```python
from build123d import *

# Parameters (mm, degrees)
SKETCH1_R                = 4
BOSS_EXTRUDE1_DEPTH      = 5
BOSS_EXTRUDE2_DEPTH      = 50
BOSS_EXTRUDE2_DEPTH_BACK = 55
SKETCH2_W                = 150
SKETCH2_H                = 5
FILLET1_R                = 25


with BuildPart() as part:
    # Sketch1 → Boss-Extrude1 (new body)
    with BuildSketch(Plane.XY):
        with BuildLine():
            Line((-366.666725266, 12.5), (-126.666725266, 12.5))
            Line((-126.666725266, 12.5), (53.333274734, 12.5))
            ThreePointArc((53.333274734, 12.5), (60.404342545, 9.571067812), (63.333274734, 2.5))
            Line((63.333274734, 2.5), (63.333274734, -2.5))
            ThreePointArc((63.333274734, -2.5), (60.404342545, -9.571067812), (53.333274734, -12.5))
            Line((53.333274734, -12.5), (-126.666725266, -12.5))
            Line((-126.666725266, -12.5), (-366.666725266, -12.5))
            ThreePointArc((-366.666725266, -12.5), (-373.737793078, -9.571067812), (-376.666725266, -2.5))
            Line((-376.666725266, -2.5), (-376.666725266, 2.5))
            ThreePointArc((-376.666725266, 2.5), (-373.737793078, 9.571067812), (-366.666725266, 12.5))
        make_face()
        with Locations(Location((53.333274734, 0, 0), (0, 0, 180))):
            Circle(SKETCH1_R, mode=Mode.SUBTRACT)
        with BuildLine():
            Line((-366.666725266, 4), (-176.666725266, 4))
            ThreePointArc((-176.666725266, 4), (-172.666725266, 0), (-176.666725266, -4))
            Line((-176.666725266, -4), (-366.666725266, -4))
            ThreePointArc((-366.666725266, -4), (-370.666725266, 0), (-366.666725266, 4))
        make_face(mode=Mode.SUBTRACT)
    extrude(amount=BOSS_EXTRUDE1_DEPTH)

    # Sketch2 → Boss-Extrude2 (add, two sides: drawn at the far end of the back side and taken through both)
    with BuildSketch(Plane.XY.offset(5).offset(-BOSS_EXTRUDE2_DEPTH_BACK)):
        with Locations((-89.389943781, 10)):
            Rectangle(SKETCH2_W, SKETCH2_H)
    extrude(amount=BOSS_EXTRUDE2_DEPTH + BOSS_EXTRUDE2_DEPTH_BACK)

    # Fillet1
    fillet1_edges = [part.edges().sort_by_distance(p)[0] for p in [
        (-14.389943781, 10, -50),
        (-164.389943781, 10, -50),
        (-164.389943781, 10, 55),
        (-14.389943781, 10, 55),
    ]]
    fillet(fillet1_edges, radius=FILLET1_R)


solid = part.part
```
The listing builds one solid part. Answer for the finished solid, in the listing's coordinates (mm). A direction names the side the tool comes from. Give positions to 0.01 mm unless a question says otherwise; leave off trailing zeros. Write each loop counter-clockwise with the first axis right and the second up, starting at its lowest first coordinate (ties: lowest second). Pieces come first, ordered by that corner, then holes. Notation, with made-up numbers: (36.5, 88) -> (87.5, 88) arc R19 ccw to (87.5, 123) -> close; hole circle Ø11 at (76, -37). An arc over 180 degrees is marked (long way). Write item = value, one per line. Start each with the question number.
1) Each of these flat-tipped pins is pushed along its axis until it touches: pin 1 (5 mm diameter, centred on x = -86, z = 42.5, fed in from -Y); pin 2 (2 mm diameter, centred on y = 5, z = 5, fed in from -X); pin 3 (1.5 mm diameter, centred on y = 11, z = 14.5, fed in from -X). Where does it stop, or does it pass through?
2) The part is cut by section D-D, the plane x = -31. Determine the outline of the cut face in (y, z), and give its area (4 significant figures).
3) Determine the mould class of faces 1 (the face through (-154, 0, 0)), 2 (the face through (60.326, 9.648, 2.465)), 3 (the face through (56.51, 2.43, 2.46)), 4 (the face through (-157.261, 10.035, -42.482)) for opening direction X: +X half, -X half, draft (parallel to the pull), parting line (faces both ways), or undercut.
4) Straight lines are drawn through the part: line 1 along Z through (x, y) = (40.5, 3.25); line 2 along Y through (x, z) = (-17, -8); line 3 along X through (y, z) = (9.75, -45). For each, find the intervals that lie inside material, in ascending order.
5) Which of the six approach directions +Z, -Z, +X, -X, +Y, -Y give full straight-line access (tool end or side, diameter ignored) to faces 5 (the face through (-90, 7.5, 30)), 6 (the face through (-90, 7.5, -25)), 7 (the face through (-21.519, 10.035, 47.482))?
6) The part is cut by section C-C, the plane z = -41. Determine the outline of the cut face in (x, y).
7) The part is cut by section A-A, the plane x = -241.5. Determine the outline of the cut face in (y, z).
8) The part is cut by section B-B, the plane x = -77.5. Determine the outline of the cut face in (y, z).
Solutions:
q1.pin_1 = 7.5
q1.pin_2 = -376.55
q1.pin_3 = -164.39
q2.outline = (-12.5, 0) -> (7.5, 0) -> (7.5, -48.55) -> (12.5, -48.55) -> (12.5, 53.55) -> (7.5, 53.55) -> (7.5, 5) -> (-12.5, 5) -> close
q2.area = 610.5 mm²
q3.face_1 = draft
q3.face_2 = +X half
q3.face_3 = undercut
q3.face_4 = -X half
q4.line_1 = 0 to 5
q4.line_2 = 7.5 to 12.5
q4.line_3 = -154.39 to -24.39
q5.face_5 = +Z, +X, -X, -Y
q5.face_6 = -Z, +X, -X, -Y
q5.face_7 = +Z, +X, +Y, -Y
q6.outline = (-158.6, 7.5) -> (-20.18, 7.5) -> (-20.18, 12.5) -> (-158.6, 12.5) -> close
q7.outline = (-12.5, 0) -> (-4, 0) -> (-4, 5) -> (-12.5, 5) -> close; (4, 0) -> (12.5, 0) -> (12.5, 5) -> (4, 5) -> close
q8.outline = (-12.5, 0) -> (7.5, 0) -> (7.5, -50) -> (12.5, -50) -> (12.5, 55) -> (7.5, 55) -> (7.5, 5) -> (-12.5, 5) -> close
